from build123d import *

# Parameters (mm, degrees)
F0_W     = 216
F0_H     = 128
F0_R     = 2.5
F1_DEPTH = 5
F2_W     = 216
F2_H     = 128
F2_W_2   = 208
F2_H_2   = 120
F3_DEPTH = 45


with BuildPart() as f1:
    # F0 (on Front) → F1 (new body)
    with BuildSketch(Plane.XZ):
        with Locations((-7.728394, 22.219788)):
            Rectangle(F0_W, F0_H)
        with Locations((-103.228394, -29.278811)):
            Circle(F0_R, mode=Mode.SUBTRACT)
        with Locations((87.771606, -29.280212)):
            Circle(F0_R, mode=Mode.SUBTRACT)
        with Locations((-103.228394, 73.719788)):
            Circle(F0_R, mode=Mode.SUBTRACT)
        with Locations((87.771606, 73.719788)):
            Circle(F0_R, mode=Mode.SUBTRACT)
    extrude(amount=F1_DEPTH)

    # F2 (on face) → F3 (join)
    with BuildSketch(Plane(origin=(0, 0, 0), x_dir=(-1, 0, 0), z_dir=(0, 1, 0))):
        with Locations((7.728394, 22.219788)):
            Rectangle(F2_W, F2_H)
        with Locations((7.728394, 22.219788)):
            Rectangle(F2_W_2, F2_H_2, mode=Mode.SUBTRACT)
    extrude(amount=F3_DEPTH)


solid = f1.part
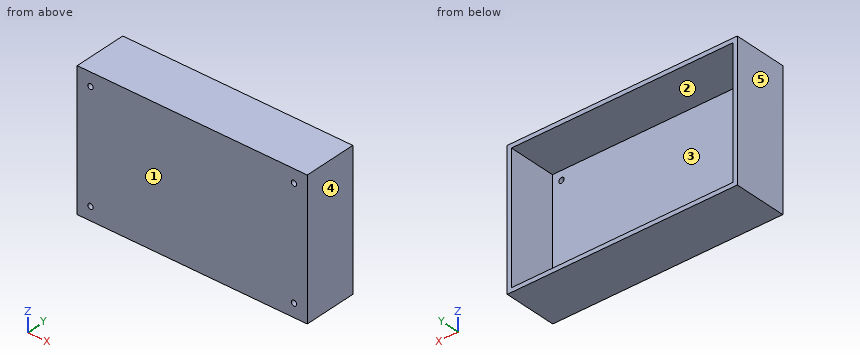
Part model, mm, in its own coordinate system. Face numbers are marked on the shaded views. A direction names the side the tool comes from. Coordinates: 2 decimals unless noted, no trailing zeros. Order: outer loops, then holes, each group sorted by start corner. A loop starts at its lowest first (then second) coordinate and runs counter-clockwise, first axis right, second up. Notation, with made-up numbers: M -28,-29.5 L -18,-29.5 A25 ccw -18,7.5 Z; hole C -15,37.25 d10. An arc over 180 degrees is marked long. Use a Markdown table: item, result.
(1) Cut at C-C on z = -13.5. Write the cut outline in (x, y).
A:
| item | result |
|---|---|
| outline | M -115.73,-5 L 100.27,-5 L 100.27,45 L 96.27,45 L 96.27,0 L -111.73,0 L -111.73,45 L -115.73,45 Z |
(2) Flat gauge pin, fed straight in: pin 1 (6.5 mm diameter, centred on x = -103.23, z = -29.28, fed in from +Y). Where does the tip first touch, or does it go through?
A:
| item | result |
|---|---|
| pin 1 | stops at y = 0 |
(3) Cut at A-A on x = 62. Write the cut outline in (y, z), then the cut area to 3 significant figures.
A:
| item | result |
|---|---|
| outline | M -5,-41.78 L 45,-41.78 L 45,-37.78 L 0,-37.78 L 0,82.22 L 45,82.22 L 45,86.22 L -5,86.22 Z |
| area | 1,000 mm^2 |
(4) Tool access for the marked faces 1 and 2: list every direction of +Z, -Z, +X, -X, +Y, -Y with a clear straight run to the whole face (end or side of a thin tool).
A:
| item | result |
|---|---|
| face 1 | +Z, -Z, +X, -X, -Y |
| face 2 | +Y |
(5) Probe L1, parallel to X at y = 12, z = 44.5; L2, parallel to Z at x = -34, y = 38; L3, parallel to Y at x = -78, z = 59.5. List the from-to ranges inside material, lowest first.
A:
| item | result |
|---|---|
| L1 | x = -115.73 to -111.73, 96.27 to 100.27 |
| L2 | z = -41.78 to -37.78, 82.22 to 86.22 |
| L3 | y = -5 to 0 |
(6) Cut at B-B on y = 10. Write the cut outline in (x, z), then the cut area to 3 significant figures.
A:
| item | result |
|---|---|
| outline | M -115.73,-41.78 L 100.27,-41.78 L 100.27,86.22 L -115.73,86.22 Z; hole M -111.73,-37.78 L 96.27,-37.78 L 96.27,82.22 L -111.73,82.22 Z |
| area | 2,690 mm^2 |
(7) Pull direction X, two halves, no side cores. Call the marked faces 3, 4 and 5: released by +X, released by -X, zero draft, split by the parting line, or undercut.
A:
| item | result |
|---|---|
| face 3 | undercut |
| face 4 | released by +X |
| face 5 | released by -X |
